For this review, take the finished solid that the model builds, in its own axes (mm). Face numbers are marked on the shaded views. A direction names the side the tool comes from. Coordinates: 2 decimals unless noted, no trailing zeros. Loops run counter-clockwise (first coordinate to the right, second up) from the corner with the lowest first, then second, coordinate; pieces in that order, holes last. Notation, with made-up numbers: (-9, -6.5) - (40, -6.5) arc R12 ccw to (40, 8.5) - close; hole circle Ø8 at (-22, -32). An arc over 180 degrees is marked (long way). Answer as a JSON object with one key per item and string values. Group by question number.
Item 1: We need section A-A (x = 66). Give the boundary of the cut face in (y, z), then the cut area to 3 significant figures.
Item 2: We need section C-C (z = 10). Give the boundary of the cut face in (x, y), then the cut area to 3 significant figures.
Item 3: Clearance check with flat-ended pins moving along their axes: pin 1 (0.8 mm diameter, centred on x = 64.5, z = 40.5, fed in from +Y); pin 2 (3 mm diameter, centred on y = 6, z = -6, fed in from -X); pin 3 (5.5 mm diameter, centred on x = -4.5, z = -2.5, fed in from +Y); pin 4 (7.5 mm diameter, centred on x = 46, y = 13.2, fed in from +Z). State where each tip first meets the part, or that it passes through.
Item 4: We need section B-B (x = 36). Give the boundary of the cut face in (y, z), then the cut area to 3 significant figures.
Item 5: Tool access review of the marked faces 4 and 5: name each direction out of +Z, -Z, +X, -X, +Y, -Y from which nothing blocks a thin tool from reaching the whole face with its end or side.
Item 6: Mouldability with a two-part tool opening along X and no side actions: class the marked faces 1, 2 and 3 as released by +X, released by -X, zero draft, split by the parting line, or undercut.
Item 7: To check wall thickness, follow line 1 (Z direction, x = -75, y = 6); line 2 (X direction, y = 1.5, z = -7); line 3 (X direction, y = 11.5, z = 34.5). State the ranges of each line that lie inside material, in increasing order.
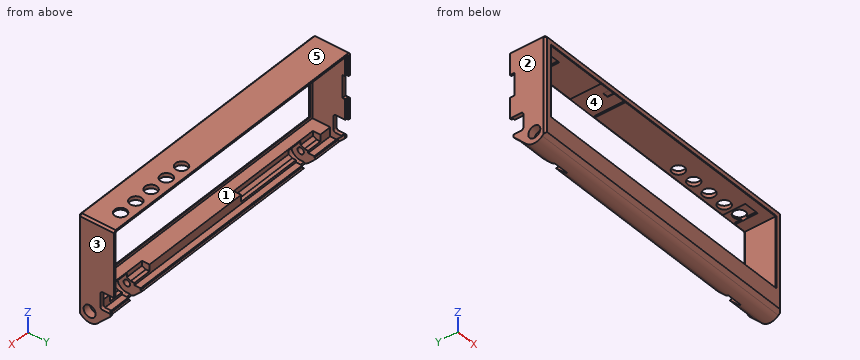
from build123d import *

# Parameters (mm, degrees)
PAD_DEPTH            = 77.4
SKETCH002_W          = 40
SKETCH002_H          = 150
POCKET_DEPTH         = 18.501
SKETCH005_W          = 38
SKETCH005_H          = 148
POCKET003_DEPTH      = 0.501
SKETCH021_W          = 40.8
SKETCH021_H          = 150.8
POCKET018_DEPTH      = 18.501
SKETCH003_W          = 4
SKETCH003_H          = 8
SKETCH003_H_2        = 10
SKETCH003_H_3        = 36
SKETCH003_W_2        = 1.4
POCKET001_DEPTH      = 13.001
CHAMFER_1_SIZE2      = 1
CHAMFER_1_SIZE       = 2
CHAMFER_2_SIZE2      = 1
CHAMFER_2_SIZE       = 2
CHAMFER_3_SIZE2      = 1
CHAMFER_3_SIZE       = 2
CHAMFER_4_SIZE2      = 1
CHAMFER_4_SIZE       = 2
SKETCH004_W          = 4.8
SKETCH004_H          = 150
POCKET002_DEPTH      = 9.001
SKETCH022_W          = 5.2
SKETCH022_H          = 150.8
POCKET019_DEPTH      = 9.001
POCKET009_DEPTH      = 8
SKETCH013_R          = 1.7
POCKET010_DEPTH      = 40
SKETCH014_R          = 3.2
POCKET011_DEPTH      = 4
SKETCH006_W          = 1
SKETCH006_H          = 16
POCKET004_DEPTH      = 17.1
SKETCH020_W          = 5
SKETCH020_H          = 3
POCKET017_DEPTH      = 0.2
POCKET005_DEPTH      = 77.401
POCKET005_DEPTH_BACK = 77.401
SKETCH016_W          = 5
SKETCH016_H          = 12
POCKET012_DEPTH      = 10
SKETCH008_W          = 40
SKETCH008_H          = 152.8
POCKET006_DEPTH      = 1.001
SKETCH023_W          = 30
SKETCH023_H          = 170
POCKET020_DEPTH      = 2
POCKET007_DEPTH      = 76.4
SKETCH010_R          = 3.2
POCKET008_DEPTH      = 2.401
CHAMFER001_SIZE      = 1
CHAMFER002_SIZE      = 0.5


with BuildPart() as part:
    # Sketch001 → Pad (new body, symmetric)
    with BuildSketch(Plane.YZ):
        with BuildLine():
            Line((19, -1.485281), (19, 42.4))
            Line((0, 42.4), (19, 42.4))
            Line((0, 42.4), (0, 0))
            Line((0, 0), (0, -8.485281))
            Line((0, -8.485281), (1.757359, -10.242641))
            ThreePointArc((1.757359, -10.242641), (6, -12), (10.242641, -10.242641))
            Line((10.242641, -10.242641), (19, -1.485281))
        make_face()
    extrude(amount=PAD_DEPTH, both=True)

    # Sketch002 (on Face3 of Pad) → Pocket (cut, through all)
    with BuildSketch(Plane(origin=(0, 0.5, 0), x_dir=(0, 0, -1), z_dir=(0, -1, 0))):
        with Locations((-20, 0)):
            Rectangle(SKETCH002_W, SKETCH002_H)
    extrude(amount=-POCKET_DEPTH, mode=Mode.SUBTRACT)

    # Sketch005 (on Face14 of Pocket) → Pocket003 (cut, through all)
    with BuildSketch(Plane.ZX.offset(0.5)):
        with Locations((20, 0)):
            Rectangle(SKETCH005_W, SKETCH005_H)
    extrude(amount=-POCKET003_DEPTH, mode=Mode.SUBTRACT)

    # Sketch021 (on Face14 of Pocket) → Pocket018 (cut, through all)
    with BuildSketch(Plane.ZX.offset(0.5)):
        with Locations((20, 0)):
            Rectangle(SKETCH021_W, SKETCH021_H)
    extrude(amount=POCKET018_DEPTH, mode=Mode.SUBTRACT)

    # Sketch003 (on Face3 of Pad) → Pocket001 (cut, through all)
    with BuildSketch(Plane(origin=(0, 6, 0), x_dir=(0, 0, -1), z_dir=(0, -1, 0))):
        with Locations((2, 65)):
            Rectangle(SKETCH003_W, SKETCH003_H)
        with Locations((2, 48)):
            Rectangle(SKETCH003_W, SKETCH003_H_2)
        with Locations((2, -35)):
            Rectangle(SKETCH003_W, SKETCH003_H_3)
        with Locations((2, -65)):
            Rectangle(SKETCH003_W, SKETCH003_H)
        with Locations((-40.7, 65)):
            Rectangle(SKETCH003_W_2, SKETCH003_H)
        with Locations((-40.7, -65)):
            Rectangle(SKETCH003_W_2, SKETCH003_H)
    extrude(amount=-POCKET001_DEPTH, mode=Mode.SUBTRACT)

    # Chamfer 1
    chamfer_1_edges = [part.edges().sort_by_distance(p)[0] for p in [
        (65, 6, -4),
    ]]
    chamfer_1_side = part.faces().sort_by_distance((65, 11.242641, -4))[0]
    chamfer(chamfer_1_edges, length=CHAMFER_1_SIZE, length2=CHAMFER_1_SIZE2, reference=chamfer_1_side)

    # Chamfer 2
    chamfer_2_edges = [part.edges().sort_by_distance(p)[0] for p in [
        (48, 6, -4),
    ]]
    chamfer_2_side = part.faces().sort_by_distance((48, 11.242641, -4))[0]
    chamfer(chamfer_2_edges, length=CHAMFER_2_SIZE, length2=CHAMFER_2_SIZE2, reference=chamfer_2_side)

    # Chamfer 3
    chamfer_3_edges = [part.edges().sort_by_distance(p)[0] for p in [
        (-35, 6, -4),
    ]]
    chamfer_3_side = part.faces().sort_by_distance((-35, 11.242641, -4))[0]
    chamfer(chamfer_3_edges, length=CHAMFER_3_SIZE, length2=CHAMFER_3_SIZE2, reference=chamfer_3_side)

    # Chamfer 4
    chamfer_4_edges = [part.edges().sort_by_distance(p)[0] for p in [
        (-65, 6, -4),
    ]]
    chamfer_4_side = part.faces().sort_by_distance((-65, 11.242641, -4))[0]
    chamfer(chamfer_4_edges, length=CHAMFER_4_SIZE, length2=CHAMFER_4_SIZE2, reference=chamfer_4_side)

    # Sketch004 (on Face3 of Pad) → Pocket002 (cut, through all)
    with BuildSketch(Plane(origin=(0, 10, 0), x_dir=(0, 0, -1), z_dir=(0, -1, 0))):
        with Locations((2.4, 0)):
            Rectangle(SKETCH004_W, SKETCH004_H)
    extrude(amount=-POCKET002_DEPTH, mode=Mode.SUBTRACT)

    # Sketch022 (on Face4 of Pocket002) → Pocket019 (cut, through all)
    with BuildSketch(Plane.ZX.offset(10)):
        with Locations((-2.6, 0)):
            Rectangle(SKETCH022_W, SKETCH022_H)
    extrude(amount=POCKET019_DEPTH, mode=Mode.SUBTRACT)

    # Sketch011 (on Face33 of Pocket001) → Pocket009 (cut)
    with BuildSketch(Plane.YZ.offset(61)):
        with BuildLine():
            ThreePointArc((6, -1), (1, -6), (6, -11))
            Line((6, -11), (7.8, -11))
            Line((7.8, -11), (8.8, -12))
            Line((8.8, -12), (21, -12))
            Line((21, 4), (21, -12))
            Line((6, 4), (21, 4))
            Line((6, -1), (6, 4))
        make_face()
    pocket009 = extrude(amount=-POCKET009_DEPTH, mode=Mode.SUBTRACT)

    # Sketch013 (on Face9 of Pad) → Pocket010 (cut)
    with BuildSketch(Plane.YZ.offset(77.4)):
        with Locations((6, -6)):
            Circle(SKETCH013_R)
    pocket010 = extrude(amount=-POCKET010_DEPTH, mode=Mode.SUBTRACT)

    # Sketch014 (on Face9 of Pad) → Pocket011 (cut)
    with BuildSketch(Plane.YZ.offset(77.4)):
        with Locations((6, -6)):
            Circle(SKETCH014_R)
    pocket011 = extrude(amount=-POCKET011_DEPTH, mode=Mode.SUBTRACT)

    # Mirrored: Pocket011, Pocket010, Pocket009 across YZ
    add(pocket011.mirror(Plane.YZ), mode=Mode.SUBTRACT)
    add(pocket010.mirror(Plane.YZ), mode=Mode.SUBTRACT)
    add(pocket009.mirror(Plane.YZ), mode=Mode.SUBTRACT)

    # Sketch006 (on Face14 of Pocket) → Pocket004 (cut)
    with BuildSketch(Plane.ZX.offset(0.9)):
        with Locations((40.9, -31)):
            Rectangle(SKETCH006_W, SKETCH006_H)
    extrude(amount=POCKET004_DEPTH, mode=Mode.SUBTRACT)

    # Sketch020 (on Face82 of Pocket004) → Pocket017 (cut)
    with BuildSketch(Plane.YX.offset(-41.4)):
        with Locations((3.4, -31)):
            Rectangle(SKETCH020_W, SKETCH020_H)
    extrude(amount=-POCKET017_DEPTH, mode=Mode.SUBTRACT)

    # Sketch007 → Pocket005 (cut, two sides)
    with BuildSketch(Plane.YZ) as pocket005_sk:
        with BuildLine():
            Line((13, 7.35), (21.8, 7.35))
            Line((21.8, 7.35), (21.8, -1.95))
            Line((21.8, -1.95), (13, -1.95))
            ThreePointArc((11.8, -0.75), (12.151472, -1.598528), (13, -1.95))
            Line((11.8, 6.15), (11.8, -0.75))
            ThreePointArc((13, 7.35), (12.151472, 6.998528), (11.8, 6.15))
        make_face()
    extrude(amount=-POCKET005_DEPTH, mode=Mode.SUBTRACT)
    extrude(pocket005_sk.sketch, amount=POCKET005_DEPTH_BACK, mode=Mode.SUBTRACT)

    # Sketch016 (on Face8 of Pad) → Pocket012 (cut)
    with BuildSketch(Plane(origin=(-77.4, 0, 0), x_dir=(0, 1, 0), z_dir=(-1, 0, 0))):
        with Locations((19.1, -24.2)):
            Rectangle(SKETCH016_W, SKETCH016_H)
    extrude(amount=-POCKET012_DEPTH, mode=Mode.SUBTRACT)

    # Sketch008 (on Face1 of Pad) → Pocket006 (cut, through all)
    with BuildSketch(Plane.ZX.offset(18)):
        with Locations((21.4, 0)):
            Rectangle(SKETCH008_W, SKETCH008_H)
    extrude(amount=POCKET006_DEPTH, mode=Mode.SUBTRACT)

    # Sketch023 (on Face1 of Pad) → Pocket020 (cut)
    with BuildSketch(Plane.ZX.offset(19)):
        with Locations((-15, 0)):
            Rectangle(SKETCH023_W, SKETCH023_H)
    extrude(amount=-POCKET020_DEPTH, mode=Mode.SUBTRACT)

    # Sketch009 → Pocket007 (cut, symmetric)
    with BuildSketch(Plane.YZ):
        Polygon((13.285281, -6.2), (23.285281, -6.2), (23.285281, 6.8), (16, -0.485281), (16, -2.485281), (13.285281, -5.2), align=None)
    extrude(amount=POCKET007_DEPTH, both=True, mode=Mode.SUBTRACT)

    # Sketch010 (on Face7 of Pocket) → Pocket008 (cut, through all)
    with BuildSketch(Plane.YX.offset(-40)):
        with Locations((13.2, 66)):
            Circle(SKETCH010_R)
        with Locations((13.2, 56)):
            Circle(SKETCH010_R)
        with Locations((13.2, 46)):
            Circle(SKETCH010_R)
        with Locations((13.2, 36)):
            Circle(SKETCH010_R)
        with Locations((13.2, 26)):
            Circle(SKETCH010_R)
    extrude(amount=-POCKET008_DEPTH, mode=Mode.SUBTRACT)

    # Chamfer001
    chamfer001_edges = [part.edges().sort_by_distance(p)[0] for p in [
        (77.4, 0, 21.2),
        (77.4, 9.5, 42.4),
        (-77.4, 0, 21.2),
        (-77.4, 9.5, 42.4),
        (0, 0, 42.4),
    ]]
    chamfer(chamfer001_edges, length=CHAMFER001_SIZE)

    # Chamfer002
    chamfer002_edges = [part.edges().sort_by_distance(p)[0] for p in [
        (-76.4, 18.5, 41.4),
        (76.4, 18.5, 41.4),
    ]]
    chamfer(chamfer002_edges, length=CHAMFER002_SIZE)


solid = part.part
Check sheet entries:
{
 "1": {"outline": "(0, -8.49) - (1.76, -10.24) arc R6 ccw to (10.24, -10.24) - (14.29, -6.2) - (13.29, -6.2) - (13.29, -5.2) - (10, -5.2) - (10, -4) - (8, -4) - (6, -3) - (6, -0.4) - (0.5, -0.4) - (0.5, 1) - (0, 1) - close; (0, 39) - (0.5, 39) - (0.5, 40.4) - (6, 40.4) - (6, 41.4) - (10, 41.4) - (10, 42.4) - (1, 42.4) - (0, 41.4) - close; (16.4, 41.4) - (19, 41.4) - (19, 42.4) - (16.4, 42.4) - close; hole circle Ø3.4 at (6, -6)", "area": "117 mm2"},
 "2": {"outline": "(-77.4, 1) - (-76.4, 0) - (-74, 0) - (-74, 0.5) - (-75.4, 0.5) - (-75.4, 18) - (-76.4, 18) - (-76.4, 19) - (-77.4, 19) - close; (74, 0) - (76.4, 0) - (77.4, 1) - (77.4, 19) - (76.4, 19) - (76.4, 18) - (75.4, 18) - (75.4, 0.5) - (74, 0.5) - close", "area": "74.4 mm2"},
 "3": {"pin 1": "stops at y = 6", "pin 2": "stops at x = -37.4", "pin 3": "stops at y = 13.29", "pin 4": "stops at z = 42.4"},
 "4": {"outline": "(0, -8.49) - (1.76, -10.24) arc R6 ccw to (10.24, -10.24) - (14.29, -6.2) - (13.29, -6.2) - (13.29, -5.2) - (10, -5.2) - (10, -0.4) - (0.5, -0.4) - (0.5, 1) - (0, 1) - close; (0, 39) - (0.5, 39) - (0.5, 40.4) - (10, 40.4) - (10, 42.4) - (1, 42.4) - (0, 41.4) - close; (16.4, 40.4) - (18, 40.4) - (18, 41.4) - (19, 41.4) - (19, 42.4) - (16.4, 42.4) - close", "area": "145 mm2"},
 "5": {"face 4": "+Y", "face 5": "+Z, +X, -X, +Y, -Y"},
 "6": {"face 1": "undercut", "face 2": "released by -X", "face 3": "released by +X"},
 "7": {"line 1": "z = -12 to -9.2, -2.8 to -0.4, 40.4 to 42.4", "line 2": "x = -77.4 to -61, -53 to 53, 61 to 77.4", "line 3": "x = -77.4 to -75.4, 75.4 to 77.4"}
}
